Check sheet for the modelled part. Datum: model origin and axes. Units: mm. A direction names the side the tool comes from. Give positions to 0.01 mm unless a question says otherwise; leave off trailing zeros. Loops run counter-clockwise (first coordinate to the right, second up) from the corner with the lowest first, then second, coordinate; pieces in that order, holes last. Notation, with made-up numbers: (43.25, 54.5) - (73.25, 54.5) arc R7 ccw to (73.25, 58.5) - close; hole circle Ø1 at (82, -19.75). An arc over 180 degrees is marked (long way). Use CSV: the item, a comma, the result in double quotes.
Autodesk Inventor part; units mm, degrees
ref_plane "Work Plane3" through (37.0477, -2.5, 47.5652) normal (0.9397, 0, 0.342) x (0, 1, 0)
ref_plane "YZ Plane" through (0, 0, 0) normal (1, 0, 0) x (0, 1, 0)
ref_plane "XZ Plane" through (0, 0, 0) normal (0, 1, 0) x (-1, 0, 0)
sketch "Sketch1" plane through (0, 0, 0) normal (0, 0, 1) x (1, 0, 0)
  circle A0 centre (0, 30) radius 8.45
  circle A1 centre (0, 30) radius 6
  arc A2 (-30, 0) -> (-15.2201, 12.4401) centre (-30, 15) ccw
  arc A3 (15.2201, 12.4401) -> (30, 0) centre (30, 15) ccw
  arc A4 (11.824, 32.0479) -> (-11.824, 32.0479) centre (0, 30) ccw
  line L0 (-11.824, 32.0479) -> (-15.2201, 12.4401)
  line L1 (11.824, 32.0479) -> (15.2201, 12.4401)
  line L2 (30, 0) -> (-30, 0)
  line L3 (-30, 0) -> (-30, -2.5)
  line L4 (-30, -2.5) -> (30, -2.5)
  line L5 (30, -2.5) -> (30, 0)
  point P0 (0, 0)
  point P1 (0, 0)
  dimension "d2" = 16.9
  dimension "d3" = 12
  dimension "d9" = 30
  dimension "d12" = 12
  dimension "d15" = 15
  dimension "d16" = 60
  dimension "d17" = 2.5
extrude "Extrusion3" add sketch "Sketch1" along normal mid plane 30 contours A2 L0 A4 L1 A3 L2
extrude "Extrusion4" add sketch "Sketch1" along normal mid plane 20 contours A0
extrude "Extrusion5" add sketch "Sketch1" against normal blind 15 contours L2 L5 L4 L3
extrude "Extrusion6" add sketch "Sketch1" along normal blind 45 contours L2 L5 L4 L3
ref_plane "Work Plane1" through (30, -2.5, 45) normal (0.9397, 0, 0.342) x (0, 1, 0)
ref_plane "Work Plane3" through (37.0477, -2.5, 47.5652) normal (0.9397, 0, 0.342) x (0, 1, 0)
sketch "Sketch5" plane through (37.0477, -2.5, 47.5652) normal (0.9397, 0, 0.342) x (0, 1, 0)
  line L0 (2.5, -28.1908) -> (2.5, -16.1908) construction
  circle A0 centre (10.5, -9.9886) radius 5.35
  circle A1 centre (10.5, -9.9886) radius 7.3 construction
  line L1 (2.5, -16.1908) -> (6.65, -16.1908)
  line L2 (6.65, -16.1908) -> (6.65, -3.7863)
  line L3 (6.65, -3.7863) -> (2.5, -3.7863)
  line L4 (2.5, -3.7863) -> (2.5, -16.1908)
  point P0 (6.65, -13.7034)
  point P1 (6.65, -6.2737)
  dimension "d46" = 12
  dimension "d47" = 10.7
  dimension "d48" = 14.6
  dimension "d49" = 8
  dimension "d51" = 1.5
extrude "Extrusion9" add sketch "Sketch5" along normal mid plane 5.5 contours A0 L2 L1 L4 L3
sketch "Sketch6" plane through (30, -2.5, -15) normal (1, 0, 0) x (0, 0, -1)
  line L0 (0, 0) -> (-60, 0)
  line L1 (0, 2.5) -> (0, 0)
  line L2 (0, 2.5) -> (-30, 2.5)
  line L3 (-30, 2.5) -> (-60, 2.5)
  line L4 (-60, 0) -> (-60, 2.5)
  point P0 (-15, 2.5)
extrude "Extrusion10" add sketch "Sketch6" along normal blind 15
sketch "Sketch7" plane through (-30, 0, 15) normal (0, 1, 0) x (1, 0, 0)
  line L0 (0, 30) -> (0, -30)
  arc A0 (67.5578, -30) -> (0, 0) centre (0, -91.0677) ccw
  line L1 (0, -30) -> (75, -30)
  line L2 (0, 0) -> (60, 0)
  arc A1 (60, 30) -> (75, -18.0474) centre (144.4517, 30) ccw
  line L3 (60, 30) -> (60, 0)
  line L4 (75, 30) -> (75, -30)
  line L5 (60, 30) -> (75, 30)
  point P0 (30, 15)
  point P1 (65.7585, -28.0666)
  point P2 (75.1694, -18.2914)
extrude "Extrusion11" cut sketch "Sketch7" against normal through all contours A0 L1 L0 | L5 L4 A1
properties part number "Support"
1. Sectioned sample at B-B, the plane x = 0. Record the boundary of the cut face in (y, z).
Completed:
outline,"(-2.5, -15) - (21.55, -15) - (21.55, -10) - (24, -10) - (24, 10) - (21.55, 10) - (21.55, 15) - (0, 15) - (0, 20.08) - (-2.5, 20.08) - close; (36, -10) - (38.45, -10) - (38.45, -15) - (42, -15) - (42, 15) - (38.45, 15) - (38.45, 10) - (36, 10) - close"
2. Scan lines: line 1 along Y through (x, z) = (0, -12); line 2 along Z through (x, y) = (-12, 0.5); line 3 along Y through (x, z) = (39.5, 24). Record each from-to range of solid material in increasing order.
Completed:
line 1,"y = -2.5 to 21.55, 38.45 to 42"
line 2,"z = -15 to 15"
line 3,"y = -2.5 to 0"
3. Release check for a two-part mould opening along Z. For faces 1 (the face through (40.45, 2.65, 38.11)), 2 (the face through (13.5, 22.38, -0.21)), 3 (the face through (42.55, 2.05, 32.34)) record: released by +Z, released by -Z, zero draft, split by the parting line, or undercut.
Completed:
face 1,"undercut"
face 2,"zero draft"
face 3,"released by -Z"
4. Sectioned sample at C-C, the plane z = 12. Record the boundary of the cut face in (x, y).
Completed:
outline,"(-30, -2.5) - (34.43, -2.5) - (34.43, 0) - (30, 0) arc R15 cw to (15.22, 12.44) - (11.82, 32.05) arc R12 ccw to (-11.82, 32.05) - (-15.22, 12.44) arc R15 cw to (-30, 0) - close; hole circle Ø16.9 at (0, 30)"
5. Set-up check for faces 4 (the face through (2, 36, -10)), 5 (the face through (2, 36, 10)), 6 (the face through (43.02, 1.58, 39.2)): record each of +Z, -Z, +X, -X, +Y, -Y from which the full face is reachable in a straight line by a thin tool's end or side.
Completed:
face 4,"-Z"
face 5,"+Z"
face 6,"+Z, +X, +Y"
6. Sectioned sample at D-D, the plane y = 30. Record the boundary of the cut face in (x, z).
Completed:
outline,"(-12.18, -15) - (-8.45, -15) - (-8.45, -10) - (-6, -10) - (-6, 10) - (-8.45, 10) - (-8.45, 15) - (-12.18, 15) - close; (6, -10) - (8.45, -10) - (8.45, -15) - (12.18, -15) - (12.18, 15) - (8.45, 15) - (8.45, 10) - (6, 10) - close"
7. Go/stop test with flat-tipped pins: pin 1 Ø10 at (y, z) = (17.5, -2.5) entering from +X; pin 2 Ø1.5 at (x, z) = (26.5, 35) entering from +Y; pin 3 Ø9.5 at (x, y) = (0, 30) entering from -Z; pin 4 Ø3 at (y, z) = (29, 14.5) entering from -X. Record where each tip stops, or that it passes through.
Completed:
pin 1,"stops at x = 15.21"
pin 2,"stops at y = 0"
pin 3,"passes through"
pin 4,"stops at x = -12.61"
8. Sectioned sample at A-A, the plane y = 34.5. Record the boundary of the cut face in (x, z).
Completed:
outline,"(-11.12, -15) - (-7.15, -15) - (-7.15, -10) - (-3.97, -10) - (-3.97, 10) - (-7.15, 10) - (-7.15, 15) - (-11.12, 15) - close; (3.97, -10) - (7.15, -10) - (7.15, -15) - (11.12, -15) - (11.12, 15) - (7.15, 15) - (7.15, 10) - (3.97, 10) - close"
